Verification items for the finished model (mm, model axes). A direction names the side the tool comes from. Coordinates: 2 decimals unless noted, no trailing zeros. Loops run counter-clockwise (first coordinate to the right, second up) from the corner with the lowest first, then second, coordinate; pieces in that order, holes last. Notation, with made-up numbers: (12.25, 27.25) -> (55.25, 27.25) arc R27 ccw to (55.25, 62.25) -> close; hole circle Ø5 at (51, 32). An arc over 180 degrees is marked (long way). Write item = value, one per line.
```python
from build123d import *

# Parameters (mm, degrees)
F0_W      = 304.8
F0_H      = 152.4
F1_DEPTH  = 19.05
F2_W      = 101.6
F2_H      = 19.05
F3_DEPTH  = 19.051
F4_W      = 19.304
F4_H      = 49.53
F5_DEPTH  = 19.051
F6_W      = 6.35
F6_H      = 6.35
F7_DEPTH  = 152.401
F9_DEPTH  = 19.051
F10_R     = 19.05
F11_DEPTH = 19.051
F12_W     = 50.8
F12_H     = 19.05
F13_DEPTH = 19.05


with BuildPart() as f1:
    # F0 (on Right) → F1 (new body)
    with BuildSketch(Plane.YZ):
        with Locations((-96.171215, -95.702616)):
            Rectangle(F0_W, F0_H)
    extrude(amount=F1_DEPTH)

    # F2 (on face) → F3 (cut, through all)
    with BuildSketch(Plane.YZ.offset(19.05)):
        with Locations((-197.771215, -162.377616)):
            Rectangle(F2_W, F2_H)
        with Locations((5.428785, -162.377616)):
            Rectangle(F2_W, F2_H)
    extrude(amount=-F3_DEPTH, mode=Mode.SUBTRACT)

    # F4 (on face) → F5 (cut, through all)
    with BuildSketch(Plane.YZ.offset(19.05)):
        with Locations((-96.171215, -86.177616)):
            Rectangle(F4_W, F4_H)
    extrude(amount=-F5_DEPTH, mode=Mode.SUBTRACT)

    # F6 (on face) → F7 (cut, through all)
    with BuildSketch(Plane.XY.offset(-19.502616)):
        with Locations((3.175, 34.003785)):
            Rectangle(F6_W, F6_H)
    extrude(amount=-F7_DEPTH, mode=Mode.SUBTRACT)

    # F8 (on face) → F9 (cut, through all)
    with BuildSketch(Plane.YZ.offset(19.05)):
        Polygon((-146.971215, -19.502616), (-248.571215, -19.502616), (-248.571215, -121.102616), align=None)
    extrude(amount=-F9_DEPTH, mode=Mode.SUBTRACT)

    # F10 (on face) → F11 (cut, through all)
    with BuildSketch(Plane.YZ.offset(19.05)):
        with Locations((-7.271215, -86.177616)):
            Circle(F10_R)
    extrude(amount=-F11_DEPTH, mode=Mode.SUBTRACT)

    # F12 (on face) → F13 (join)
    with BuildSketch(Plane(origin=(0, 0, 0), x_dir=(0, -1, 0), z_dir=(-1, 0, 0))):
        with Locations((28.099215, -9.977616)):
            Rectangle(F12_W, F12_H)
    extrude(amount=-F13_DEPTH)


solid = f1.part
```
1) Tool access check on faces 4 (the face through (10, -96, -61.413)), 5 (the face through (10, 5, -152.853)), 6 (the face through (6.35, 34, -85)). Record the directions out of +Z, -Z, +X, -X, +Y, -Y that give a thin tool (end or side, any length) a straight path to the whole face; none if there is none.
Ans:
face_4 = +X, -X
face_5 = -Z, +X, -X, +Y
face_6 = +Z, -Z, -X
2) Release check for a two-part mould opening along Y. For faces 1 (the face through (9.66, -198.48, -71.01)), 2 (the face through (0, 47, -85)), 3 (the face through (10, -105.823, -87)) record: pulls with the +Y half, pulls with the -Y half, needs draft (parallel to the pull), parting line crosses it, or undercut.
Ans:
face_1 = pulls with the -Y half
face_2 = needs draft
face_3 = undercut
3) Sectioned sample at C-C, the plane z = -100. Record the cut outline in (x, y), plus the area to 3 significant figures.
Ans:
outline = (0, -227.47) -> (19.05, -227.47) -> (19.05, -105.82) -> (0, -105.82) -> close; (0, -86.52) -> (19.05, -86.52) -> (19.05, -20.38) -> (0, -20.38) -> close; (0, 5.84) -> (19.05, 5.84) -> (19.05, 56.23) -> (0, 56.23) -> (0, 37.18) -> (6.35, 37.18) -> (6.35, 30.83) -> (0, 30.83) -> close
area = 4,500 mm2
4) Sectioned sample at B-B, the plane y = -101.5. Record the cut outline in (x, z), plus the area to 3 significant figures.
Ans:
outline = (0, -171.9) -> (19.05, -171.9) -> (19.05, -110.94) -> (0, -110.94) -> close; (0, -61.41) -> (19.05, -61.41) -> (19.05, -19.5) -> (0, -19.5) -> close
area = 1,960 mm2
5) Sectioned sample at D-D, the plane z = -39. Record the cut outline in (x, y), plus the area to 3 significant figures.
Ans:
outline = (0, -166.47) -> (19.05, -166.47) -> (19.05, 56.23) -> (0, 56.23) -> (0, 37.18) -> (6.35, 37.18) -> (6.35, 30.83) -> (0, 30.83) -> close
area = 4,200 mm2
6) Depth check by flat-ended pin: pin 1 Ø9.5 at (x, y) = (10, -114) entering from +Z; pin 2 Ø3 at (x, z) = (4.5, -83.5) entering from -Y; pin 3 Ø1.9 at (y, z) = (34, -72.5) entering from -X; pin 4 Ø23 at (y, z) = (-7.27, -86.18) entering from -X. Enter the tip coordinate at first touch or a pass-through.
Ans:
pin_1 = -19.5
pin_2 = -212.47
pin_3 = 6.35
pin_4 = through
7) Sectioned sample at A-A, the plane x = 3. Record the cut outline in (y, z), plus the area to 3 significant figures.
Ans:
outline = (-248.57, -152.85) -> (-146.97, -152.85) -> (-146.97, -171.9) -> (-45.37, -171.9) -> (-45.37, -152.85) -> (30.83, -152.85) -> (30.83, -19.5) -> (-2.7, -19.5) -> (-2.7, -0.45) -> (-53.5, -0.45) -> (-53.5, -19.5) -> (-146.97, -19.5) -> (-248.57, -121.1) -> close; (37.18, -152.85) -> (56.23, -152.85) -> (56.23, -19.5) -> (37.18, -19.5) -> close; hole (-105.82, -110.94) -> (-86.52, -110.94) -> (-86.52, -61.41) -> (-105.82, -61.41) -> close; hole circle Ø38.1 at (-7.27, -86.18)
area = 35,400 mm2
8) Material ranges on line 1 (Z direction, x = 16.25, y = -95.5); line 2 (Z direction, x = 4.75, y = -7.5); line 3 (Y direction, x = 17.25, z = -89.5), recorded low to high.
Ans:
line_1 = -171.9 to -110.94, -61.41 to -19.5
line_2 = -152.85 to -105.23, -67.13 to -0.45
line_3 = -216.97 to -105.82, -86.52 to -26.03, 11.49 to 56.23
